```python
from build123d import *

# Parameters (mm, degrees)
SKETCH2_W           = 100
SKETCH2_H           = 100
BOSS_EXTRUDE1_DEPTH = 1500
CUT_EXTRUDE1_REACH  = 1508.652
SKETCH3_R           = 25
SKETCH4_W           = 200
SKETCH4_H           = 200
BOSS_EXTRUDE2_DEPTH = 50
SKETCH5_W           = 50
SKETCH5_H           = 45
BOSS_EXTRUDE3_DEPTH = 200
FILLET1_R           = 5


with BuildPart() as part:
    # Sketch2 → Boss-Extrude1 (new body)
    with BuildSketch(Plane.XY):
        with Locations((50, 50)):
            Rectangle(SKETCH2_W, SKETCH2_H)
    extrude(amount=BOSS_EXTRUDE1_DEPTH)

    # Sketch3 → Cut-Extrude1 (cut, up to next)
    with BuildSketch(Plane.XZ, mode=Mode.PRIVATE) as cut_extrude1_sk1:
        with Locations(Location((55, 1455, 0), (0, 0, 270))):
            Circle(SKETCH3_R)
    cut_extrude1_tool1 = extrude(cut_extrude1_sk1.sketch, amount=-CUT_EXTRUDE1_REACH, mode=Mode.PRIVATE) & part.part
    add(cut_extrude1_tool1.solids().sort_by_distance((55, 0, 1455))[0], mode=Mode.SUBTRACT)

    # Sketch4 → Boss-Extrude2 (add)
    with BuildSketch(Plane(origin=(0, 0, 0), x_dir=(-1, 0, 0), z_dir=(0, 0, -1))):
        with Locations((-50, 50)):
            Rectangle(SKETCH4_W, SKETCH4_H)
    extrude(amount=-BOSS_EXTRUDE2_DEPTH)

    # Sketch5 → Boss-Extrude3 (add)
    with BuildSketch(Plane.XZ.offset(50)):
        with Locations((5, -22.5)):
            Rectangle(SKETCH5_W, SKETCH5_H)
        with Locations((95, -22.5)):
            Rectangle(SKETCH5_W, SKETCH5_H)
    extrude(amount=-BOSS_EXTRUDE3_DEPTH)

    # Fillet1
    fillet1_edges = [part.edges().sort_by_distance(p)[0] for p in [
        (30, 50, 0),
        (-20, 50, 0),
        (120, 50, 0),
        (70, 50, 0),
    ]]
    fillet(fillet1_edges, radius=FILLET1_R)


solid = part.part
```
Geometry check sheet. Reference: the model listing, model coordinates, mm. A direction names the side the tool comes from. Give positions to 0.01 mm unless a question says otherwise; leave off trailing zeros. Order: outer loops, then holes, each group sorted by start corner. A loop starts at its lowest first (then second) coordinate and runs counter-clockwise, first axis right, second up.
1. Gauge pin test, flat ends, axial feed: pin 1 Ø12.5 at (x, y) = (141.5, 39) entering from -Z; pin 2 Ø1.5 at (x, y) = (23.5, -4.5) entering from +Z; pin 3 Ø5 at (y, z) = (33.5, 216) entering from -X. Record the tip position at first contact, or that the pin passes through.
2. Release check for a two-part mould opening along X. For faces 5 (the face through (138, 51, 0)), 6 (the face through (50, 51, 0)), 7 (the face through (150, 49, 25)) record: pulls with the +X half, pulls with the -X half, needs draft (parallel to the pull), parting line crosses it, or undercut.
3. Section check B-B, the plane y = 87. Enter the section's corners in (x, z).
4. Section check C-C, the plane z = 186. Enter the section's corners in (x, y).
5. Thickness scan on L1, parallel to X at y = 79, z = 1455; L2, parallel to Z at x = 131.5, y = 11; L3, parallel to Z at x = 91.5, y = 117. Record the ranges inside material, lowest first.
6. Section check A-A, the plane z = 1455. Enter the section's corners in (x, y), and give its area (3 significant figures).
7. Access from +Z, -Z, +X, -X, +Y, -Y to the whole of each face (thin tool, end or side, straight path). Record for faces 1 (the face through (100, 49, 765)), 2 (the face through (70, 49, -25)), 3 (the face through (0, 49, 765)), 4 (the face through (49, 100, 765)).
Values follow:
1. pin 1: stops at z = 0
1. pin 2: stops at z = 50
1. pin 3: stops at x = 0
2. face 5: needs draft
2. face 6: undercut
2. face 7: pulls with the +X half
3. outline: (-50, 0) - (-25, 0) arc R5 cw to (-20, -5) - (-20, -45) - (30, -45) - (30, -5) arc R5 cw to (35, 0) - (65, 0) arc R5 cw to (70, -5) - (70, -45) - (120, -45) - (120, -5) arc R5 cw to (125, 0) - (150, 0) - (150, 50) - (100, 50) - (100, 1500) - (0, 1500) - (0, 50) - (-50, 50) - close; hole circle Ø50 at (55, 1455)
4. outline: (0, 0) - (100, 0) - (100, 100) - (0, 100) - close
5. L1: x = 0 to 30, 80 to 100
5. L2: z = 0 to 50
5. L3: z = -45 to 50
6. outline: (0, 0) - (30, 0) - (30, 100) - (0, 100) - close; (80, 0) - (100, 0) - (100, 100) - (80, 100) - close
6. area: 5,000 mm2
7. face 1: +Z, +X, +Y, -Y
7. face 2: -Z, +Y, -Y
7. face 3: +Z, -X, +Y, -Y
7. face 4: +Z, +X, -X, +Y
